Can you work these out from the model? Positions are in its coordinate system, mm. Round coordinates to 2 decimals unless told otherwise and drop trailing zeros. Order: outer loops, then holes, each group sorted by start corner. A loop starts at its lowest first (then second) coordinate and runs counter-clockwise, first axis right, second up. Notation, with made-up numbers: (42, -38) - (58, -38) arc R24 cw to (58, -21) - close; hole circle Ø3 at (24, 42.5). An arc over 180 degrees is marked (long way). Write item = value, one per line.
from build123d import *

# Parameters (mm, degrees)
EXTRUDE_1_OUTLINE_R      = 50
EXTRUDE_1_OUTLINE_R_2    = 47
EXTRUDE_1_DEPTH          = 200
CUT_EXTRUDE_1_DEPTH      = 213.132034356
CUT_EXTRUDE_1_DEPTH_BACK = 213.132034356
SKETCH_2_R               = 65


# Read off the part's stored shape, not the designer's step: Вытянуть-Тонкостенный1
with BuildPart() as part:
    # Вытянуть-Тонкостенный1 outline → Вытянуть-Тонкостенный1 (new body)
    with BuildSketch(Plane(origin=(0, 0, 0), x_dir=(1, 0, 0), z_dir=(0, 1, 0))):
        Circle(EXTRUDE_1_OUTLINE_R)
        Circle(EXTRUDE_1_OUTLINE_R_2, mode=Mode.SUBTRACT)
    extrude(amount=EXTRUDE_1_DEPTH)

    # Эскиз2 → Вырез-Вытянуть1 (cut, two sides: drawn at the far end of the back side and taken through both)
    with BuildSketch(Plane(origin=(0, 0, 0), x_dir=(1, 0, 0), z_dir=(0, -0.5735764363510444, -0.819152044288993)).offset(-CUT_EXTRUDE_1_DEPTH_BACK)):
        with Locations((0, -180)):
            Circle(SKETCH_2_R)
    extrude(amount=CUT_EXTRUDE_1_DEPTH + CUT_EXTRUDE_1_DEPTH_BACK, mode=Mode.SUBTRACT)


solid = part.part
(1) If we section it at C-C (x = 30.5): Write out the boundary of the cut face in (y, z), plus the area to 3 significant figures.
Computed:
outline = (0, -39.62) - (121.92, -39.62) - (124.63, -35.76) - (0, -35.76) - close; (0, 35.76) - (174.71, 35.76) - (177.41, 39.62) - (0, 39.62) - close
area = 1,160 mm^2
(2) Will these pins go through, and if not, where does the flat tip stop? P1, Ø10, axis at y = 83.5, z = 10.5, coming from the -X side; P2, Ø4, axis at x = 14, y = 110.5, coming from the +Z side; P3, Ø12, axis at x = -34.5, y = 49, coming from the -Z side.
Computed:
P1 = -49.7
P2 = 48.54
P3 = -41.08
(3) If I drill on line 1 (Z direction, x = 0, y = 104); line 2 (X direction, y = 70, z = 21.5), over which ranges is the centre line in solid material (lowest first)? Write a range as from..to.
Computed:
line_1 = -50..-47, 47..50
line_2 = -45.14..-41.79, 41.79..45.14
(4) If we section it at A-A (x = 43): Write out the boundary of the cut face in (y, z).
Computed:
outline = (0, -25.51) - (142.37, -25.51) - (146.95, -18.97) - (0, -18.97) - close; (0, 18.97) - (173.52, 18.97) - (178.1, 25.51) - (0, 25.51) - close
(5) If we section it at B-B (y = 66): Write out the boundary of the cut face in (x, z), plus the area to 3 significant figures.
Computed:
outline = circle Ø100 at (0, 0); hole circle Ø94 at (0, 0)
area = 914 mm^2
